Answer from the drawing. Dimensions are ordinates in mm from the lowest x, y and z of the part. Coordinates: 2 decimals unless noted, no trailing zeros. Order: outer loops, then holes, each group sorted by start corner. A loop starts at its lowest first (then second) coordinate and runs counter-clockwise, first axis right, second up. Notation, with made-up numbers: (7, 44) -> (49, 44) arc R30 ccw to (49, 77) -> close; hole circle Ø6 at (24.5, 40.5). An arc over 180 degrees is marked (long way). Answer in a Markdown table with one row per item.
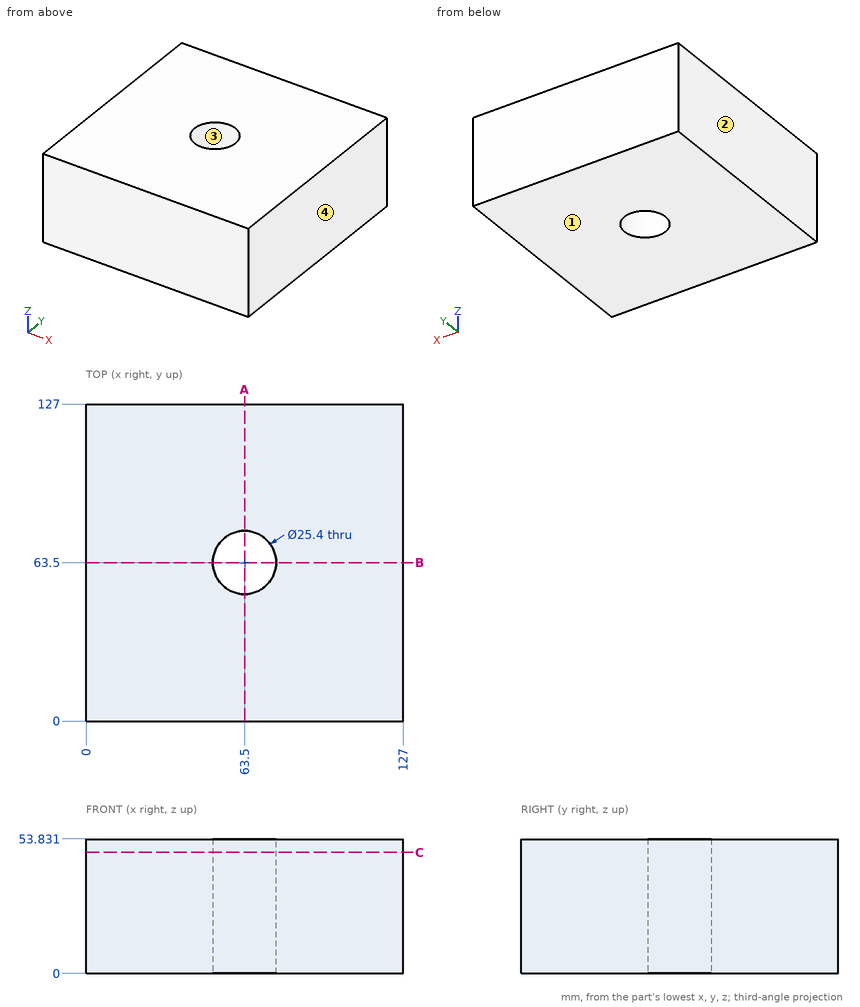
(1) Find the intervals of material crossed by line 1 along Y through (x, z) = (63.5, 27); line 2 along Y through (x, z) = (67.5, 5), in increasing order. Write a range as from..to.
Check values:
| item | result |
|---|---|
| line 1 | 0..50.8, 76.2..127 |
| line 2 | 0..51.45, 75.55..127 |
(2) A cutting plane is placed at C-C, the plane z = 48.5. Determine the outline of the cut face in (x, y), then the cut area to 3 significant figures.
Check values:
| item | result |
|---|---|
| outline | (0, 0) -> (127, 0) -> (127, 127) -> (0, 127) -> close; hole circle Ø25.4 at (63.5, 63.5) |
| area | 15,600 mm² |
(3) For a pull along X with two mould halves and no side action, classify the marked faces 1, 2, 3 and 4 as released by +X, released by -X, zero draft, split by the parting line, or undercut.
Check values:
| item | result |
|---|---|
| face 1 | zero draft |
| face 2 | released by -X |
| face 3 | undercut |
| face 4 | released by +X |
(4) A cutting plane is placed at A-A, the plane x = 63.5. Determine the outline of the cut face in (y, z), then the cut area to 3 significant figures.
Check values:
| item | result |
|---|---|
| outline | (0, 0) -> (50.8, 0) -> (50.8, 53.83) -> (0, 53.83) -> close; (76.2, 0) -> (127, 0) -> (127, 53.83) -> (76.2, 53.83) -> close |
| area | 5,470 mm² |
